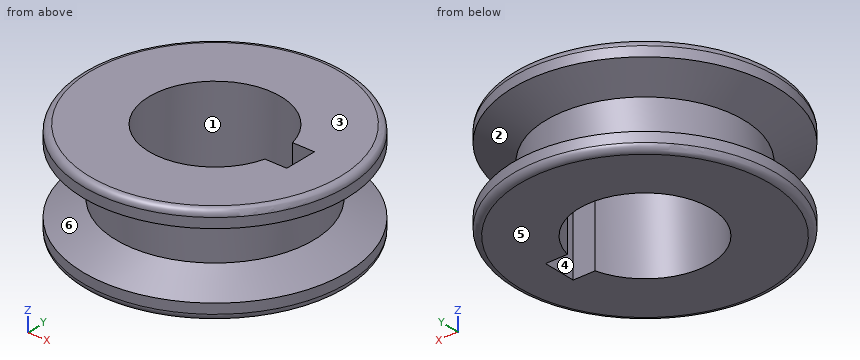
```python
from build123d import *

# Parameters (mm, degrees)
SKETCH_1_R               = 20
SKETCH_1_R_2             = 10
EXTRUDE_1_DEPTH          = 15
CUT_EXTRUDE_1_DEPTH      = 3
CUT_EXTRUDE_1_DEPTH_BACK = 10
FILLET_1_R               = 1


with BuildPart() as part:
    # 草图1 → 凸台-拉伸1 (new body)
    with BuildSketch(Plane.XY):
        Circle(SKETCH_1_R)
        Circle(SKETCH_1_R_2, mode=Mode.SUBTRACT)
    extrude(amount=EXTRUDE_1_DEPTH)

    # 草图2 → 切除-旋转1 (revolve, cut)
    with BuildSketch(Plane(origin=(0, 0, 0), x_dir=(0, 0, -1), z_dir=(1, 0, 0))):
        Polygon((-5, 15), (-2.5, 20), (-12.5, 20), (-10, 15), align=None)
    revolve(axis=Axis((0, 0, -0.75), (0, 0, 1)), mode=Mode.SUBTRACT)

    # 草图3 → 切除-拉伸1 (cut, two sides)
    with BuildSketch(Plane(origin=(10, 0, 0), x_dir=(0, 0, -1), z_dir=(1, 0, 0))) as cut_extrude_1_sk:
        with BuildLine():
            Line((-15.73557603, 2.5), (0, 2.5))
            ThreePointArc((0, 2.5), (2.5, 0), (0, -2.5))
            Line((0, -2.5), (-15.73557603, -2.5))
            ThreePointArc((-15.73557603, -2.5), (-18.23557603, 0), (-15.73557603, 2.5))
        make_face()
    extrude(amount=CUT_EXTRUDE_1_DEPTH, mode=Mode.SUBTRACT)
    extrude(cut_extrude_1_sk.sketch, amount=-CUT_EXTRUDE_1_DEPTH_BACK, mode=Mode.SUBTRACT)

    # 圆角1
    fillet_1_edges = [part.edges().sort_by_distance(p)[0] for p in [
        (-20, 0, 0),
        (-20, 0, 15),
    ]]
    fillet(fillet_1_edges, radius=FILLET_1_R)


solid = part.part
```
Model file for the job. Use its own axes, mm. Face numbers are marked on the shaded views. A direction names the side the tool comes from. Coordinates: 2 decimals unless noted, no trailing zeros. Order: outer loops, then holes, each group sorted by start corner. A loop starts at its lowest first (then second) coordinate and runs counter-clockwise, first axis right, second up. Notation, with made-up numbers: (0, 12.5) - (8, 12.5) arc R13 cw to (8, 27.5) - close; hole circle Ø1 at (12, 23). An arc over 180 degrees is marked (long way). Return JSON: item names as keys, results as strings. Group by question number.
1) Flat gauge pins, fed straight in: P1, Ø3, axis at y = 3.5, z = 3, coming from the -X side; P2, Ø8, axis at x = -11, z = 12, coming from the -Y side; P3, Ø1.7, axis at x = 11, z = 8.5, coming from the -Y side. Where does each tip first touch, or does it go through?
2) Tool access for the marked faces 4, 5 and 6: list every direction of +Z, -Z, +X, -X, +Y, -Y with a clear straight run to the whole face (end or side of a thin tool).
3) Saw through at B-B, the plane y = 0. Write the cut outline in (x, z), plus the area to 3 significant figures.
4) Mould opens along Y. For the marked faces 1, 2 and 3 say: released by +Y, released by -Y, zero draft, split by the parting line, or undercut.
5) Saw through at A-A, the plane x = 0. Write the cut outline in (y, z), plus the area to 3 significant figures.
6) Saw through at C-C, the plane z = 8. Write the cut outline in (x, y).
7) Saw through at D-D, the plane z = 4.25. Write the cut outline in (x, y).
8) Probe line 1 (X direction, y = 0, z = 6.25); line 2 (X direction, y = 0, z = 11); line 3 (Y direction, x = -7.5, z = 10.25). List the from-to ranges inside material, lowest first. Write a range as from..to.
Values found:
{
 "1": {"P1": "stops at x = -19.89", "P2": "stops at y = -18.72", "P3": "stops at y = -11.04"},
 "2": {"face 4": "+Z, -Z", "face 5": "-Z, +X, -X, +Y, -Y", "face 6": "none"},
 "3": {"outline": "(-20, 1) arc R1 ccw to (-19, 0) - (-10, 0) - (-10, 15) - (-19, 15) arc R1 ccw to (-20, 14) - (-20, 12.5) - (-15, 10) - (-15, 5) - (-20, 2.5) - close; (13, 0) - (19, 0) arc R1 ccw to (20, 1) - (20, 2.5) - (15, 5) - (15, 10) - (20, 12.5) - (20, 14) arc R1 ccw to (19, 15) - (13, 15) - close", "area": "179 mm²"},
 "4": {"face 1": "undercut", "face 2": "split by the parting line", "face 3": "zero draft"},
 "5": {"outline": "(-20, 1) arc R1 ccw to (-19, 0) - (-10, 0) - (-10, 15) - (-19, 15) arc R1 ccw to (-20, 14) - (-20, 12.5) - (-15, 10) - (-15, 5) - (-20, 2.5) - close; (10, 0) - (19, 0) arc R1 ccw to (20, 1) - (20, 2.5) - (15, 5) - (15, 10) - (20, 12.5) - (20, 14) arc R1 ccw to (19, 15) - (10, 15) - close", "area": "224 mm²"},
 "6": {"outline": "circle Ø30 at (0, 0); hole (9.68, -2.5) - (13, -2.5) - (13, 2.5) - (9.68, 2.5) arc R10 ccw (long way) to start"},
 "7": {"outline": "circle Ø33 at (0, 0); hole (9.68, -2.5) - (13, -2.5) - (13, 2.5) - (9.68, 2.5) arc R10 ccw (long way) to start"},
 "8": {"line 1": "x = -15..-10, 13..15", "line 2": "x = -17..-10, 13..17", "line 3": "y = -13.56..-6.61, 6.61..13.56"}
}
